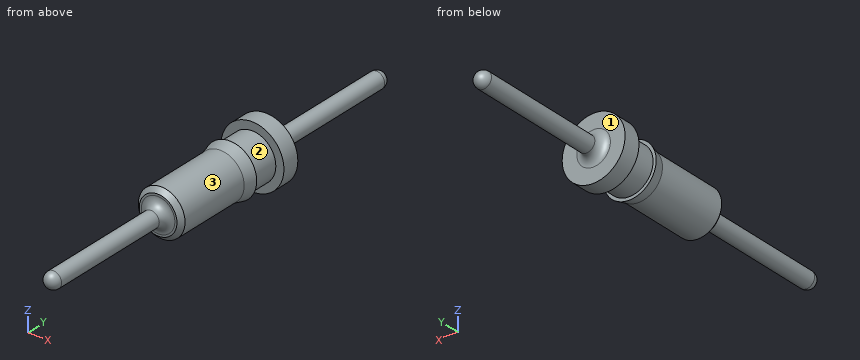
```python
from build123d import *

# Parameters (mm, degrees)
DOME1_FACE_RADIUS = 0.235
DOME1_HEIGHT      = 0.235
DOME2_FACE_RADIUS = 0.235
DOME2_HEIGHT      = 0.235
FILLET1_R         = 0.25


with BuildPart() as part:
    # Sketch1 → Revolve1 (revolve)
    with BuildSketch(Plane.XY):
        Polygon((0, 0), (0, 11.64), (0.235, 11.64), (0.235, 7.67), (0.91, 7.67), (0.91, 7.17), (0.675, 7.17), (0.675, 6.37), (0.765, 6.37), (0.675, 6.03), (0.675, 3.9), (0.545, 3.77), (0.235, 3.77), (0.235, 0), align=None)
    revolve(axis=Axis((0, 0, 0), (0, 1, 0)))

    # Dome1: a dome of height H over a round flat face of radius A is a cap of a sphere of radius (A * A + H * H) / (2 * H)
    dome1_r = (DOME1_FACE_RADIUS * DOME1_FACE_RADIUS + DOME1_HEIGHT * DOME1_HEIGHT) / (2 * DOME1_HEIGHT)
    dome1_base = Plane((0, 11.64, 0), z_dir=(0, 1, 0))
    with Locations(dome1_base.offset(DOME1_HEIGHT - dome1_r)):
        dome1_ball = Sphere(dome1_r, mode=Mode.PRIVATE)
    add(split(dome1_ball, bisect_by=dome1_base, keep=Keep.TOP, mode=Mode.PRIVATE))

    # Dome2: a dome of height H over a round flat face of radius A is a cap of a sphere of radius (A * A + H * H) / (2 * H)
    dome2_r = (DOME2_FACE_RADIUS * DOME2_FACE_RADIUS + DOME2_HEIGHT * DOME2_HEIGHT) / (2 * DOME2_HEIGHT)
    dome2_base = Plane((0, 0, 0), z_dir=(0, -1, 0))
    with Locations(dome2_base.offset(DOME2_HEIGHT - dome2_r)):
        dome2_ball = Sphere(dome2_r, mode=Mode.PRIVATE)
    add(split(dome2_ball, bisect_by=dome2_base, keep=Keep.TOP, mode=Mode.PRIVATE))

    # Fillet1
    fillet1_edges = [part.edges().sort_by_distance(p)[0] for p in [
        (-0.235, 7.67, 0),
        (-0.235, 3.77, 0),
    ]]
    fillet(fillet1_edges, radius=FILLET1_R)


solid = part.part
```
CAD build for the part. Positions are in the model's coordinates, mm. Face numbers are marked on the shaded views. Coordinates: 2 decimals unless noted, no trailing zeros. Order: outer loops, then holes, each group sorted by start corner. A loop starts at its lowest first (then second) coordinate and runs counter-clockwise, first axis right, second up. Notation, with made-up numbers: M 46.5,64 L 51.5,64 A17 ccw 51.5,94 Z; hole C 15,30.5 d6. An arc over 180 degrees is marked long. Write each question's results on one line, items separated by ' | '. Start each with the question number.
Q1. Cut at B-B (z = 0). List the corners of the cut face in (x, y) (3 decimals), then the cut area to 3 significant figures.
Q2. Cut at A-A (x = 0). List the corners of the cut face in (y, z) (3 decimals).
Q3. Pull direction Y, two halves, no side cores. Call the marked faces 1, 2 and 3: +Y half, -Y half, draft (parallel to the pull), parting line (faces both ways), or undercut.
Q4. Cut at C-C (y = 10.5). List the corners of the cut face in (x, z) (3 decimals), then the cut area to 3 significant figures.
Q5. Drill centre lines: probe 1 along Y at (x, z) = (-0.35, -0.4); probe 2 along Z at (x, y) = (-0.4, 4.25); probe 3 along X at (y, z) = (2, 0.1). Where is each one in solid material? Low to high. Write a range as from..to.
Q6. Flat gauge pin, fed straight in: P1, Ø1, axis at x = 0.5, y = 6, coming from the +Z side. Where does the tip first touch, or does it go through?
Q7. Cut at D-D (y = 6.5). List the corners of the cut face in (x, z) (3 decimals).
Found:
1) outline: M -0.91,7.17 L -0.675,7.17 L -0.675,6.37 L -0.765,6.37 L -0.675,6.03 L -0.675,3.9 L -0.545,3.77 L -0.485,3.77 A0.25 cw -0.235,3.52 L -0.235,0 A0.235 ccw 0.235,0 L 0.235,3.52 A0.25 cw 0.485,3.77 L 0.545,3.77 L 0.675,3.9 L 0.675,6.03 L 0.765,6.37 L 0.675,6.37 L 0.675,7.17 L 0.91,7.17 L 0.91,7.67 L 0.485,7.67 A0.25 cw 0.235,7.92 L 0.235,11.64 A0.235 ccw -0.235,11.64 L -0.235,7.92 A0.25 cw -0.485,7.67 L -0.91,7.67 Z | area: 9.38 mm²
2) outline: M 0,-0.235 L 3.52,-0.235 A0.25 cw 3.77,-0.485 L 3.77,-0.545 L 3.9,-0.675 L 6.03,-0.675 L 6.37,-0.765 L 6.37,-0.675 L 7.17,-0.675 L 7.17,-0.91 L 7.67,-0.91 L 7.67,-0.485 A0.25 cw 7.92,-0.235 L 11.64,-0.235 A0.235 ccw 11.64,0.235 L 7.92,0.235 A0.25 cw 7.67,0.485 L 7.67,0.91 L 7.17,0.91 L 7.17,0.675 L 6.37,0.675 L 6.37,0.765 L 6.03,0.675 L 3.9,0.675 L 3.77,0.545 L 3.77,0.485 A0.25 cw 3.52,0.235 L 0,0.235 A0.235 ccw Z
3) face 1: +Y half | face 2: undercut | face 3: draft
4) outline: C 0,0 d0.47 | area: 0.173 mm²
5) probe 1: 3.77..7.67 | probe 2: -0.54..0.54 | probe 3: -0.21..0.21
6) P1: z = 0.75
7) outline: C 0,0 d1.35
